from build123d import *

# Parameters (mm, degrees)
F0_W     = 30
F0_H     = 3
F1_DEPTH = 4
F3_DEPTH = 25
F4_R     = 0.3


with BuildPart() as f1:
    # F0 (on Top) → F1 (new body)
    with BuildSketch(Plane.XY):
        with Locations((15, -1.5)):
            Rectangle(F0_W, F0_H)
    extrude(amount=F1_DEPTH)

    # F2 (on face) → F3 (cut)
    with BuildSketch(Plane.XZ.offset(3)):
        Polygon((0, 4), (0, 0), (30, 4), align=None)
    extrude(amount=-F3_DEPTH, mode=Mode.SUBTRACT)

    # F4
    f4_edges = [f1.edges().sort_by_distance(p)[0] for p in [
        (0, -1.5, 0),
    ]]
    fillet(f4_edges, radius=F4_R)


solid = f1.part
Can you work these out from the model? Positions are in its coordinate system, mm. Round coordinates to 2 decimals unless told otherwise and drop trailing zeros. Order: outer loops, then holes, each group sorted by start corner. A loop starts at its lowest first (then second) coordinate and runs counter-clockwise, first axis right, second up. Notation, with made-up numbers: (83, 24) -> (91, 24) arc R31 ccw to (91, 59) -> close; hole circle Ø7 at (-27.5, 78). An arc over 180 degrees is marked (long way). Write each question's results on one line, items separated by ' | '. Start each with the question number.
Item 1: If we section it at A-A, the plane x = 15.75: Write out the boundary of the cut face in (y, z).
Item 2: Please list where these lines run through material, in increasing order: L1, parallel to Z at x = 26.75, y = -2.6; L2, parallel to Z at x = 15, y = -2.85; L3, parallel to X at y = -0.5, z = 0.45.
Item 3: If we section it at B-B, the plane z = 1.6: Write out the boundary of the cut face in (x, y).
Results:
1) outline: (-3, 0) -> (0, 0) -> (0, 2.1) -> (-3, 2.1) -> close
2) L1: z = 0 to 3.57 | L2: z = 0 to 2 | L3: x = 4.26 to 30
3) outline: (12, -3) -> (30, -3) -> (30, 0) -> (12, 0) -> close
